CAD build for the part. Positions are in the model's coordinates, mm. A direction names the side the tool comes from. Give positions to 0.01 mm unless a question says otherwise; leave off trailing zeros. Loops run counter-clockwise (first coordinate to the right, second up) from the corner with the lowest first, then second, coordinate; pieces in that order, holes last. Notation, with made-up numbers: M 60.25,76 L 69.25,76 A18 cw 69.25,100 Z; hole C -37.75,5.5 d8. An arc over 180 degrees is marked long. Answer as CSV lines item,"result".
from build123d import *

# Parameters (mm, degrees)
SKETCH_1_R          = 59.1
SKETCH_1_R_2        = 1.6
EXTRUDE_1_DEPTH     = 3
SKETCH_2_R          = 2.1
CUT_EXTRUDE_1_DEPTH = 104.064494371
SKETCH_3_R          = 3.1
CUT_EXTRUDE_2_DEPTH = 1
CHAMFER_1_SIZE      = 0.2


with BuildPart() as part:
    # 草图1 → 凸台-拉伸1 (new body)
    with BuildSketch(Plane.XY):
        with BuildLine():
            Line((62.3, -78), (-53.9, -78))
            ThreePointArc((-53.9, -78), (-57.435533906, -76.535533906), (-58.9, -73))
            Line((-58.9, -73), (-58.9, 73))
            ThreePointArc((-58.9, 73), (-57.435533906, 76.535533906), (-53.9, 78))
            Line((-53.9, 78), (62.3, 78))
            ThreePointArc((62.3, 78), (65.835533906, 76.535533906), (67.3, 73))
            Line((67.3, 73), (67.3, -73))
            ThreePointArc((67.3, -73), (65.835533906, -76.535533906), (62.3, -78))
        make_face()
        with Locations((4, 0)):
            Circle(SKETCH_1_R, mode=Mode.SUBTRACT)
        with Locations((58.493442579, 70.964337058)):
            Circle(SKETCH_1_R_2, mode=Mode.SUBTRACT)
        with Locations((-53.705008218, 73.348219362)):
            Circle(SKETCH_1_R_2, mode=Mode.SUBTRACT)
        with Locations(Location((58.493442579, -70.964337058, 0), (0, 0, 180))):
            Circle(SKETCH_1_R_2, mode=Mode.SUBTRACT)
        with Locations(Location((-53.705008218, -73.348219362, 0), (0, 0, 180))):
            Circle(SKETCH_1_R_2, mode=Mode.SUBTRACT)
    extrude(amount=EXTRUDE_1_DEPTH)

    # 草图2 → 切除-拉伸1 (cut, through all)
    with BuildSketch(Plane.XY.offset(3)):
        with Locations((4, -65.65)):
            Circle(SKETCH_2_R)
        with Locations((4, 65.65)):
            Circle(SKETCH_2_R)
    extrude(amount=-CUT_EXTRUDE_1_DEPTH, mode=Mode.SUBTRACT)

    # 草图3 → 切除-拉伸2 (cut)
    with BuildSketch(Plane.XY.offset(3)):
        with Locations((58.493442579, -70.964337058)):
            Circle(SKETCH_3_R)
        with Locations((-53.705008218, -73.348219362)):
            Circle(SKETCH_3_R)
        with Locations(Location((-53.705008218, 73.348219362, 0), (0, 0, 180))):
            Circle(SKETCH_3_R)
        with Locations(Location((58.493442579, 70.964337058, 0), (0, 0, 180))):
            Circle(SKETCH_3_R)
    extrude(amount=-CUT_EXTRUDE_2_DEPTH, mode=Mode.SUBTRACT)

    # 倒角1
    chamfer_1_edges = [part.edges().sort_by_distance(p)[0] for p in [
        (4.2, 78, 0),
        (65.835533906, 76.535533906, 0),
        (67.3, 0, 0),
        (65.835533906, -76.535533906, 0),
        (65.835533906, 76.535533906, 3),
        (4.2, 78, 3),
        (-57.435533906, 76.535533906, 3),
        (-55.1, 0, 0),
        (-55.1, 0, 3),
        (-58.9, 0, 3),
        (56.893442579, 70.964337058, 0),
        (-57.435533906, -76.535533906, 3),
        (60.093442579, -70.964337058, 0),
        (4.2, -78, 3),
        (-55.305008218, 73.348219362, 0),
        (-52.105008218, -73.348219362, 0),
        (65.835533906, -76.535533906, 3),
        (1.9, -65.65, 0),
        (1.9, -65.65, 3),
        (1.9, 65.65, 0),
        (1.9, 65.65, 3),
        (61.593442579, 70.964337058, 3),
        (-50.605008218, 73.348219362, 3),
        (-56.805008218, -73.348219362, 3),
        (55.393442579, -70.964337058, 3),
        (4.2, -78, 0),
        (67.3, 0, 3),
        (-57.435533906, -76.535533906, 0),
        (-58.9, 0, 0),
        (-57.435533906, 76.535533906, 0),
    ]]
    chamfer(chamfer_1_edges, length=CHAMFER_1_SIZE)


solid = part.part
1) Drill centre lines: line 1 (Y direction, x = 4, z = 1); line 2 (X direction, y = 51, z = 1.1); line 3 (Y direction, x = -1, z = 0.3). Where is each one in solid material? Low to high. Write a range as from..to.
Answer below:
line 1,"y = -78..-67.75, -63.55..-59.1, 59.1..63.55, 67.75..78"
line 2,"x = -58.9..-25.86, 33.86..67.3"
line 3,"y = -78..-58.89, 58.89..78"
2) Mould opens along Y. For faces 1 (the face through (33, 53, 0)), 2 (the face through (-57.47, 76.5, 1.48)), 3 (the face through (-55, 75, 2)) say: +Y half, -Y half, draft (parallel to the pull), parting line (faces both ways), or undercut.
Answer below:
face 1,"draft"
face 2,"+Y half"
face 3,"undercut"
3) Band-saw the part on B-B on x = 4. Give the number of separate pieces and of enclosed holes in the cut face, and give its area (3 significant figures).
Answer below:
separate pieces,"4"
enclosed holes,"0"
area,"87.9 mm^2"
4) Flat gauge pins, fed straight in: pin 1 (3 mm diameter, centred on x = 57.5, y = 70, fed in from +Z); pin 2 (4 mm diameter, centred on x = 4, y = -65.65, fed in from -Z); pin 3 (3.5 mm diameter, centred on x = -53.71, y = 73.35, fed in from -Z). Where does each tip first touch, or does it go through?
Answer below:
pin 1,"stops at z = 2"
pin 2,"passes through"
pin 3,"stops at z = 0.04"
5) Which spindle directions (+Z, -Z, +X, -X, +Y, -Y) get a long thin tool onto all of the face, cutting with end or side? Do faces 4 (the face through (3.727, -63.568, 1.518)), 5 (the face through (-56.8, -73.2, 2.4)). Say none if no direction does.
Answer below:
face 4,"+Z, -Z"
face 5,"+Z"
6) Band-saw the part on C-C on y = 0. Give the cut face in (x, z).
Answer below:
outline,"M -58.9,0.2 L -58.7,0 L -55.3,0 L -55.1,0.2 L -55.1,2.8 L -55.3,3 L -58.7,3 L -58.9,2.8 Z; M 63.1,0.2 L 63.3,0 L 67.1,0 L 67.3,0.2 L 67.3,2.8 L 67.1,3 L 63.3,3 L 63.1,2.8 Z"
7) Band-saw the part on A-A on y = -65.65. Give the cut face in (x, z).
Answer below:
outline,"M -58.9,0.2 L -58.7,0 L 1.7,0 L 1.9,0.2 L 1.9,2.8 L 1.7,3 L -58.7,3 L -58.9,2.8 Z; M 6.1,0.2 L 6.3,0 L 67.1,0 L 67.3,0.2 L 67.3,2.8 L 67.1,3 L 6.3,3 L 6.1,2.8 Z"
